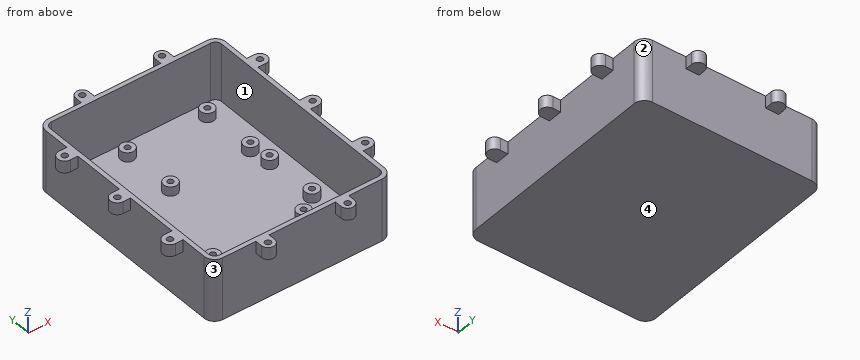
```python
from build123d import *

# Parameters (mm, degrees)
SKETCH1_W                 = 165.1
SKETCH1_H                 = 203.2
BOSS_EXTRUDE1_DEPTH       = 57.15
FILLET1_R                 = 9.525
SHELL1_T                  = -4
SKETCH2_R                 = 6.35
BOSS_EXTRUDE2_DEPTH       = 8.5
SKETCH3_R                 = 2.625
CUT_EXTRUDE1_DEPTH        = 5
SKETCH2_3_R               = 6.35
BOSS_EXTRUDE6_DEPTH       = 8.5
SKETCH13_R                = 2.625
CUT_EXTRUDE5_DEPTH        = 7
SKETCH4_R                 = 6.5
SKETCH4_R_2               = 2.75
BOSS_EXTRUDE3_DEPTH       = 11
CUT_EXTRUDE2_START        = -8
SKETCH4_6_R               = 2.75
CUT_EXTRUDE2_DEPTH        = 160.04398366
LPATTERN1_COUNT           = 2
LPATTERN1_PITCH           = 61.214
LPATTERN1_COUNT_DIR2      = 2
LPATTERN1_PITCH_DIR2      = 61.214
MIRROR1_COPY_1_SKETCH_R   = 6.5
MIRROR1_COPY_1_SKETCH_R_2 = 2.75
MIRROR1_COPY_1_DEPTH      = 11
MIRROR1_COPY_2_SKETCH_R   = 6.5
MIRROR1_COPY_2_SKETCH_R_2 = 2.75
MIRROR1_COPY_2_DEPTH      = 11
MIRROR1_COPY_3_SKETCH_R   = 6.5
MIRROR1_COPY_3_SKETCH_R_2 = 2.75
MIRROR1_COPY_3_DEPTH      = 11
MIRROR1_START             = -8
MIRROR1_COPY_4_SKETCH_R   = 2.75
MIRROR1_COPY_4_DEPTH      = 160.04398366
MIRROR1_COPY_5_SKETCH_R   = 2.75
MIRROR1_COPY_5_DEPTH      = 160.04398366
MIRROR1_COPY_6_SKETCH_R   = 2.75
MIRROR1_COPY_6_DEPTH      = 160.04398366
SKETCH12_R                = 6
SKETCH12_R_2              = 2.75
BOSS_EXTRUDE5_DEPTH       = 11
SKETCH12_3_R              = 2.75
CUT_EXTRUDE3_DEPTH        = 8


with BuildPart() as part:
    # Sketch1 → Boss-Extrude1 (new body)
    with BuildSketch(Plane.XY):
        Rectangle(SKETCH1_W, SKETCH1_H)
    extrude(amount=BOSS_EXTRUDE1_DEPTH)

    # Fillet1
    fillet1_edges = [part.edges().sort_by_distance(p)[0] for p in [
        (82.55, -101.6, 28.575),
        (-82.55, -101.6, 28.575),
        (-82.55, 101.6, 28.575),
        (82.55, 101.6, 28.575),
    ]]
    fillet(fillet1_edges, radius=FILLET1_R)

    # Shell1
    shell1_openings = [part.faces().sort_by_distance(p)[0] for p in [
        (0, 0, 57.15),
    ]]
    offset(amount=SHELL1_T, openings=shell1_openings, kind=Kind.INTERSECTION)

    # Sketch2 → Boss-Extrude2 (add)
    with BuildSketch(Plane.XY.offset(4)):
        with Locations((-41.6, -50.279)):
            Circle(SKETCH2_R)
        with Locations((-41.6, -88.279)):
            Circle(SKETCH2_R)
        with Locations((41.6, -88.279)):
            Circle(SKETCH2_R)
        with Locations((41.6, -50.279)):
            Circle(SKETCH2_R)
    extrude(amount=BOSS_EXTRUDE2_DEPTH)

    # Sketch3 → Cut-Extrude1 (cut)
    with BuildSketch(Plane.XY.offset(12.5)):
        with Locations((-41.6, -50.279)):
            Circle(SKETCH3_R)
        with Locations((-41.6, -88.279)):
            Circle(SKETCH3_R)
        with Locations((41.6, -88.279)):
            Circle(SKETCH3_R)
        with Locations((41.6, -50.279)):
            Circle(SKETCH3_R)
    extrude(amount=-CUT_EXTRUDE1_DEPTH, mode=Mode.SUBTRACT)

    # Sketch2_3 → Boss-Extrude6 (add)
    with BuildSketch(Plane.XY.offset(4)):
        with Locations((-60.516, -35.221)):
            Circle(SKETCH2_3_R)
        with Locations((-60.516, 14.011)):
            Circle(SKETCH2_3_R)
        with Locations((61.150666667, -35.221)):
            Circle(SKETCH2_3_R)
        with Locations((61.150666667, 14.011)):
            Circle(SKETCH2_3_R)
        with Locations((-13.83, 34.245)):
            Circle(SKETCH2_3_R)
        with Locations((-70.58, 34.245)):
            Circle(SKETCH2_3_R)
        with Locations((-70.58, 84.245)):
            Circle(SKETCH2_3_R)
        with Locations((-13.83, 84.245)):
            Circle(SKETCH2_3_R)
        with Locations((59.42, 84.245)):
            Circle(SKETCH2_3_R)
        with Locations((59.42, 34.245)):
            Circle(SKETCH2_3_R)
    extrude(amount=BOSS_EXTRUDE6_DEPTH)

    # Sketch13 → Cut-Extrude5 (cut)
    with BuildSketch(Plane.XY.offset(12.5)):
        with Locations((-60.516, -35.221)):
            Circle(SKETCH13_R)
        with Locations((61.150666667, -35.221)):
            Circle(SKETCH13_R)
        with Locations((61.150666667, 14.011)):
            Circle(SKETCH13_R)
        with Locations((-60.516, 14.011)):
            Circle(SKETCH13_R)
        with Locations((-13.83, 34.245)):
            Circle(SKETCH13_R)
        with Locations((-70.58, 34.245)):
            Circle(SKETCH13_R)
        with Locations((59.42, 34.245)):
            Circle(SKETCH13_R)
        with Locations((59.42, 84.245)):
            Circle(SKETCH13_R)
        with Locations((-13.83, 84.245)):
            Circle(SKETCH13_R)
        with Locations((-70.58, 84.245)):
            Circle(SKETCH13_R)
    extrude(amount=-CUT_EXTRUDE5_DEPTH, mode=Mode.SUBTRACT)

    # Sketch4 → Boss-Extrude3 (add)
    with BuildSketch(Plane.XY.offset(57.15)):
        with BuildLine():
            Line((-82.55, -6.5), (-82.55, 6.5))
            Line((-82.55, 6.5), (-89.55, 6.5))
            ThreePointArc((-89.55, 6.5), (-84.953805922, 4.596194078), (-83.05, 0))
            ThreePointArc((-83.05, 0), (-84.953805922, -4.596194078), (-89.55, -6.5))
            Line((-89.55, -6.5), (-82.55, -6.5))
        make_face()
        with Locations((-89.55, 0)):
            Circle(SKETCH4_R)
        with Locations((-89.55, 0)):
            Circle(SKETCH4_R_2)
    boss_extrude3 = extrude(amount=-BOSS_EXTRUDE3_DEPTH)

    # Sketch4_6 → Cut-Extrude2 (cut)
    with BuildSketch(Plane.XY.offset(57.15).offset(CUT_EXTRUDE2_START)):
        with Locations(Location((-89.55, 0, 0), (0, 0, 180))):
            Circle(SKETCH4_6_R)
    cut_extrude2 = extrude(amount=CUT_EXTRUDE2_DEPTH, mode=Mode.SUBTRACT)

    # LPattern1: Boss-Extrude3, Cut-Extrude2 2 × 2
    with Locations(*[Vector(0, 1, 0) * (i * LPATTERN1_PITCH) + Vector(0, -1, 0) * (j * LPATTERN1_PITCH_DIR2) for i in range(LPATTERN1_COUNT) for j in range(LPATTERN1_COUNT_DIR2) if (i, j) != (0, 0)]):
        add(boss_extrude3)
        add(cut_extrude2, mode=Mode.SUBTRACT)

    # Mirror1: Boss-Extrude3, Cut-Extrude2 across plane
    add(boss_extrude3.mirror(Plane(origin=(0, 0, 0), x_dir=(0, 0, 1), z_dir=(1, 0, 0))))
    add(cut_extrude2.mirror(Plane(origin=(0, 0, 0), x_dir=(0, 0, 1), z_dir=(1, 0, 0))), mode=Mode.SUBTRACT)

    # Mirror1 copy 1 sketch → Mirror1 copy 1 (add)
    with BuildSketch(Plane(origin=(0, -61.214, 57.15), x_dir=(-1, 0, 0), z_dir=(0, 0, 1))):
        with BuildLine():
            Line((-82.55, 6.5), (-82.55, -6.5))
            Line((-82.55, -6.5), (-89.55, -6.5))
            ThreePointArc((-89.55, -6.5), (-84.953805922, -4.596194078), (-83.05, 0))
            ThreePointArc((-83.05, 0), (-84.953805922, 4.596194078), (-89.55, 6.5))
            Line((-89.55, 6.5), (-82.55, 6.5))
        make_face()
        with Locations((-89.55, 0)):
            Circle(MIRROR1_COPY_1_SKETCH_R)
        with Locations((-89.55, 0)):
            Circle(MIRROR1_COPY_1_SKETCH_R_2)
    extrude(amount=-MIRROR1_COPY_1_DEPTH)

    # Mirror1 copy 2 sketch → Mirror1 copy 2 (add)
    with BuildSketch(Plane(origin=(0, 61.214, 57.15), x_dir=(-1, 0, 0), z_dir=(0, 0, 1))):
        with BuildLine():
            Line((-82.55, 6.5), (-82.55, -6.5))
            Line((-82.55, -6.5), (-89.55, -6.5))
            ThreePointArc((-89.55, -6.5), (-84.953805922, -4.596194078), (-83.05, 0))
            ThreePointArc((-83.05, 0), (-84.953805922, 4.596194078), (-89.55, 6.5))
            Line((-89.55, 6.5), (-82.55, 6.5))
        make_face()
        with Locations((-89.55, 0)):
            Circle(MIRROR1_COPY_2_SKETCH_R)
        with Locations((-89.55, 0)):
            Circle(MIRROR1_COPY_2_SKETCH_R_2)
    extrude(amount=-MIRROR1_COPY_2_DEPTH)

    # Mirror1 copy 3 sketch → Mirror1 copy 3 (add)
    with BuildSketch(Plane(origin=(0, 0, 57.15), x_dir=(-1, 0, 0), z_dir=(0, 0, 1))):
        with BuildLine():
            Line((-82.55, 6.5), (-82.55, -6.5))
            Line((-82.55, -6.5), (-89.55, -6.5))
            ThreePointArc((-89.55, -6.5), (-84.953805922, -4.596194078), (-83.05, 0))
            ThreePointArc((-83.05, 0), (-84.953805922, 4.596194078), (-89.55, 6.5))
            Line((-89.55, 6.5), (-82.55, 6.5))
        make_face()
        with Locations((-89.55, 0)):
            Circle(MIRROR1_COPY_3_SKETCH_R)
        with Locations((-89.55, 0)):
            Circle(MIRROR1_COPY_3_SKETCH_R_2)
    extrude(amount=-MIRROR1_COPY_3_DEPTH)

    # Mirror1 copy 4 sketch → Mirror1 copy 4 (cut)
    with BuildSketch(Plane(origin=(0, -61.214, 57.15), x_dir=(-1, 0, 0), z_dir=(0, 0, 1)).offset(MIRROR1_START)):
        with Locations((-89.55, 0)):
            Circle(MIRROR1_COPY_4_SKETCH_R)
    extrude(amount=MIRROR1_COPY_4_DEPTH, mode=Mode.SUBTRACT)

    # Mirror1 copy 5 sketch → Mirror1 copy 5 (cut)
    with BuildSketch(Plane(origin=(0, 61.214, 57.15), x_dir=(-1, 0, 0), z_dir=(0, 0, 1)).offset(MIRROR1_START)):
        with Locations((-89.55, 0)):
            Circle(MIRROR1_COPY_5_SKETCH_R)
    extrude(amount=MIRROR1_COPY_5_DEPTH, mode=Mode.SUBTRACT)

    # Mirror1 copy 6 sketch → Mirror1 copy 6 (cut)
    with BuildSketch(Plane(origin=(0, 0, 57.15), x_dir=(-1, 0, 0), z_dir=(0, 0, 1)).offset(MIRROR1_START)):
        with Locations((-89.55, 0)):
            Circle(MIRROR1_COPY_6_SKETCH_R)
    extrude(amount=MIRROR1_COPY_6_DEPTH, mode=Mode.SUBTRACT)

    # Sketch12 → Boss-Extrude5 (add)
    # profile 1 of 6: a face of its own
    with BuildSketch(Plane.XY.offset(57.15)):
        with Locations((-36.5125, -107.95)):
            Circle(SKETCH12_R)
        with Locations((-36.5125, -107.95)):
            Circle(SKETCH12_R_2, mode=Mode.SUBTRACT)
    # profile 2 of 6: a face of its own
    with BuildSketch(Plane.XY.offset(57.15)):
        with BuildLine():
            Line((-36.5125, -101.6), (-42.5125, -101.6))
            Line((-42.5125, -101.6), (-42.5125, -107.95))
            ThreePointArc((-42.5125, -107.95), (-36.5125, -101.95), (-30.5125, -107.95))
            Line((-30.5125, -107.95), (-30.5125, -101.6))
            Line((-30.5125, -101.6), (-36.5125, -101.6))
        make_face()
    # profile 3 of 6: a face of its own
    with BuildSketch(Plane.XY.offset(57.15)):
        with BuildLine():
            Line((42.5125, -101.6), (30.5125, -101.6))
            Line((30.5125, -101.6), (30.5125, -107.95))
            ThreePointArc((30.5125, -107.95), (36.5125, -101.95), (42.5125, -107.95))
            Line((42.5125, -107.95), (42.5125, -101.6))
        make_face()
    # profile 4 of 6: a face of its own
    with BuildSketch(Plane.XY.offset(57.15)):
        with Locations((36.5125, -107.95)):
            Circle(SKETCH12_R)
        with Locations((36.5125, -107.95)):
            Circle(SKETCH12_R_2, mode=Mode.SUBTRACT)
    # profile 5 of 6: a face of its own
    with BuildSketch(Plane.XY.offset(57.15)):
        with Locations((36.5125, -107.95)):
            Circle(SKETCH12_R_2)
    # profile 6 of 6: a face of its own
    with BuildSketch(Plane.XY.offset(57.15)):
        with Locations((-36.5125, -107.95)):
            Circle(SKETCH12_R_2)
    boss_extrude5 = extrude(amount=-BOSS_EXTRUDE5_DEPTH)

    # Sketch12_3 → Cut-Extrude3 (cut)
    with BuildSketch(Plane.XY.offset(57.15)):
        with Locations((-36.5125, -107.95)):
            Circle(SKETCH12_3_R)
        with Locations((36.5125, -107.95)):
            Circle(SKETCH12_3_R)
    cut_extrude3 = extrude(amount=-CUT_EXTRUDE3_DEPTH, mode=Mode.SUBTRACT)

    # Mirror2: Boss-Extrude5, Cut-Extrude3 across plane
    add(boss_extrude5.mirror(Plane.ZX))
    add(cut_extrude3.mirror(Plane.ZX), mode=Mode.SUBTRACT)


solid = part.part
```
Design review of the part built by this model. Coordinates are the model's own, in mm. Face numbers are marked on the shaded views. Give positions to 0.01 mm unless a question says otherwise; leave off trailing zeros. Write each loop counter-clockwise with the first axis right and the second up, starting at its lowest first coordinate (ties: lowest second). Pieces come first, ordered by that corner, then holes.
(1) Add section B-B (z = 16). Give the boundary of the cut face in (x, y) (3 decimals), and give its area (3 significant figures).
Checked values:
outline: (-82.55, -92.075) arc R9.525 ccw to (-73.025, -101.6) - (73.025, -101.6) arc R9.525 ccw to (82.55, -92.075) - (82.55, 92.075) arc R9.525 ccw to (73.025, 101.6) - (-73.025, 101.6) arc R9.525 ccw to (-82.55, 92.075) - close; hole (-78.55, -92.075) arc R5.525 ccw to (-73.025, -97.6) - (73.025, -97.6) arc R5.525 ccw to (78.55, -92.075) - (78.55, 92.075) arc R5.525 ccw to (73.025, 97.6) - (-73.025, 97.6) arc R5.525 ccw to (-78.55, 92.075) - close
area: 2,830 mm2
(2) Add section D-D (x = -70.58). Give the boundary of the cut face in (y, z) (3 decimals).
Checked values:
outline: (-101.6, 0) - (101.6, 0) - (101.6, 57.15) - (97.6, 57.15) - (97.6, 4) - (90.595, 4) - (90.595, 12.5) - (86.87, 12.5) - (86.87, 5.5) - (81.62, 5.5) - (81.62, 12.5) - (77.895, 12.5) - (77.895, 4) - (40.595, 4) - (40.595, 12.5) - (36.87, 12.5) - (36.87, 5.5) - (31.62, 5.5) - (31.62, 12.5) - (27.895, 12.5) - (27.895, 4) - (-97.6, 4) - (-97.6, 57.15) - (-101.6, 57.15) - close
(3) Add section A-A (y = 0). Give the boundary of the cut face in (x, z).
Checked values:
outline: (-96.05, 46.15) - (-82.55, 46.15) - (-82.55, 0) - (82.55, 0) - (82.55, 46.15) - (96.05, 46.15) - (96.05, 57.15) - (92.3, 57.15) - (92.3, 49.15) - (86.8, 49.15) - (86.8, 57.15) - (78.55, 57.15) - (78.55, 4) - (-78.55, 4) - (-78.55, 57.15) - (-86.8, 57.15) - (-86.8, 49.15) - (-92.3, 49.15) - (-92.3, 57.15) - (-96.05, 57.15) - close
(4) Wall thickness on line 1 along Y through (x, z) = (-89, 53); line 2 along Y through (x, z) = (-41.5, 10); line 3 along X through (y, z) = (-70, 22.5): over which ranges is each line inside the solid? List them lowest first.
Checked values:
line 1: y = -67.71 to -63.91, -58.52 to -54.71, -6.5 to -2.69, 2.69 to 6.5, 54.71 to 58.52, 63.91 to 67.71
line 2: y = -101.6 to -97.6, -94.63 to -90.9, -85.66 to -81.93, -56.63 to -52.9, -47.66 to -43.93, 97.6 to 101.6
line 3: x = -82.55 to -78.55, 78.55 to 82.55
(5) Clearance check with flat-ended pins moving along their axes: pin 1 Ø8 at (y, z) = (77.5, 25.5) entering from +X; pin 2 Ø5 at (x, y) = (-7.5, 53) entering from +Z; pin 3 Ø12 at (x, z) = (55, 26.5) entering from +Y. State where each tip first meets the part, or that it passes through.
Checked values:
pin 1: stops at x = 82.55
pin 2: stops at z = 4
pin 3: stops at y = 101.6
(6) Add section C-C (x = 13.5). Give the boundary of the cut face in (y, z), and give its area (3 significant figures).
Checked values:
outline: (-101.6, 0) - (101.6, 0) - (101.6, 57.15) - (97.6, 57.15) - (97.6, 4) - (-97.6, 4) - (-97.6, 57.15) - (-101.6, 57.15) - close
area: 1,240 mm2
(7) Mouldability with a two-part tool opening along Y and no side actions: class the marked faces 1, 2, 3 and 4 as +Y half, -Y half, draft (parallel to the pull), parting line (faces both ways), or undercut.
Checked values:
face 1: undercut
face 2: +Y half
face 3: -Y half
face 4: draft
